from build123d import *

# Parameters (mm, degrees)
F0_W     = 160
F0_H     = 240
F0_R     = 3.25
F1_DEPTH = 6.35


# Not quite as in the source:
# - a length typed as a fraction of an inch, garbled in the dataset ("3 / 203.2 mm" for 3/8 in), is restored


with BuildPart() as f1:
    # F0 (on Top) → F1 (new body)
    with BuildSketch(Plane.XY):
        Rectangle(F0_W, F0_H)
        with Locations((-60, -100)):
            Circle(F0_R, mode=Mode.SUBTRACT)
        with Locations((-20, -100)):
            Circle(F0_R, mode=Mode.SUBTRACT)
        with Locations((-60, -60)):
            Circle(F0_R, mode=Mode.SUBTRACT)
        with Locations((-60, -20)):
            Circle(F0_R, mode=Mode.SUBTRACT)
        with Locations((-20, -60)):
            Circle(F0_R, mode=Mode.SUBTRACT)
        with Locations((-20, -20)):
            Circle(F0_R, mode=Mode.SUBTRACT)
        with Locations((20, -100)):
            Circle(F0_R, mode=Mode.SUBTRACT)
        with Locations((60, -100)):
            Circle(F0_R, mode=Mode.SUBTRACT)
        with Locations((20, -60)):
            Circle(F0_R, mode=Mode.SUBTRACT)
        with Locations((20, -20)):
            Circle(F0_R, mode=Mode.SUBTRACT)
        with Locations((60, -60)):
            Circle(F0_R, mode=Mode.SUBTRACT)
        with Locations((60, -20)):
            Circle(F0_R, mode=Mode.SUBTRACT)
        with Locations((-60, 20)):
            Circle(F0_R, mode=Mode.SUBTRACT)
        with Locations((-20, 20)):
            Circle(F0_R, mode=Mode.SUBTRACT)
        with Locations((-60, 60)):
            Circle(F0_R, mode=Mode.SUBTRACT)
        with Locations((-60, 100)):
            Circle(F0_R, mode=Mode.SUBTRACT)
        with Locations((-20, 60)):
            Circle(F0_R, mode=Mode.SUBTRACT)
        with Locations((-20, 100)):
            Circle(F0_R, mode=Mode.SUBTRACT)
        with Locations((20, 20)):
            Circle(F0_R, mode=Mode.SUBTRACT)
        with Locations((60, 20)):
            Circle(F0_R, mode=Mode.SUBTRACT)
        with Locations((20, 60)):
            Circle(F0_R, mode=Mode.SUBTRACT)
        with Locations((20, 100)):
            Circle(F0_R, mode=Mode.SUBTRACT)
        with Locations((60, 60)):
            Circle(F0_R, mode=Mode.SUBTRACT)
        with Locations((60, 100)):
            Circle(F0_R, mode=Mode.SUBTRACT)
    extrude(amount=F1_DEPTH)


solid = f1.part
Verification items for the finished model (mm, model axes). Round coordinates to 2 decimals unless told otherwise and drop trailing zeros. Loops run counter-clockwise (first coordinate to the right, second up) from the corner with the lowest first, then second, coordinate; pieces in that order, holes last. Notation, with made-up numbers: M 33,-34.5 L 42,-34.5 A20 ccw 42,-4.5 Z; hole C -1,27 d4. An arc over 180 degrees is marked long. Write each question's results on one line, items separated by ' | '.
1) Section check B-B on z = 1.5. State how many separate pieces and enclosed holes the cut face has, then the cut area to 3 significant figures.
Checks:
separate pieces: 1 | enclosed holes: 24 | area: 37,600 mm2
2) Section check A-A on x = -20. Record the boundary of the cut face in (y, z).
Checks:
outline: M -120,0 L -103.25,0 L -103.25,6.35 L -120,6.35 Z; M -96.75,0 L -63.25,0 L -63.25,6.35 L -96.75,6.35 Z; M -56.75,0 L -23.25,0 L -23.25,6.35 L -56.75,6.35 Z; M -16.75,0 L 16.75,0 L 16.75,6.35 L -16.75,6.35 Z; M 23.25,0 L 56.75,0 L 56.75,6.35 L 23.25,6.35 Z; M 63.25,0 L 96.75,0 L 96.75,6.35 L 63.25,6.35 Z; M 103.25,0 L 120,0 L 120,6.35 L 103.25,6.35 Z
3) Scan lines: L1, parallel to X at y = 57, z = 0.75; L2, parallel to X at y = 21, z = 5. Record each from-to range of solid material in increasing order. Write a range as from..to.
Checks:
L1: x = -80..-61.25, -58.75..-21.25, -18.75..18.75, 21.25..58.75, 61.25..80 | L2: x = -80..-63.09, -56.91..-23.09, -16.91..16.91, 23.09..56.91, 63.09..80
4) Gauge pin test, flat end, axial feed: P1, Ø5, axis at x = 60, y = -20, coming from the -Z side. Record the tip position at first contact, or that the pin passes through.
Checks:
P1: passes through
5) Mould release check, pull along Y, two halves, no side actions. Record for faces 1 (the cylindrical face through (-60.705, 96.827, 3.131)), 2 (the cylindrical face through (59.295, -103.173, 3.131)), 3 (the flat face through (-1, 2, 0)), 4 (the flat face through (-1, -120, 3)): released by +Y, released by -Y, zero draft, split by the parting line, or undercut.
Checks:
face 1: undercut | face 2: undercut | face 3: zero draft | face 4: released by -Y
6) Section check C-C on y = -20. Record the boundary of the cut face in (x, z).
Checks:
outline: M -80,0 L -63.25,0 L -63.25,6.35 L -80,6.35 Z; M -56.75,0 L -23.25,0 L -23.25,6.35 L -56.75,6.35 Z; M -16.75,0 L 16.75,0 L 16.75,6.35 L -16.75,6.35 Z; M 23.25,0 L 56.75,0 L 56.75,6.35 L 23.25,6.35 Z; M 63.25,0 L 80,0 L 80,6.35 L 63.25,6.35 Z
7) Section check D-D on x = 20.5. Record the boundary of the cut face in (y, z), then the cut area to 3 significant figures.
Checks:
outline: M -120,0 L -103.21,0 L -103.21,6.35 L -120,6.35 Z; M -96.79,0 L -63.21,0 L -63.21,6.35 L -96.79,6.35 Z; M -56.79,0 L -23.21,0 L -23.21,6.35 L -56.79,6.35 Z; M -16.79,0 L 16.79,0 L 16.79,6.35 L -16.79,6.35 Z; M 23.21,0 L 56.79,0 L 56.79,6.35 L 23.21,6.35 Z; M 63.21,0 L 96.79,0 L 96.79,6.35 L 63.21,6.35 Z; M 103.21,0 L 120,0 L 120,6.35 L 103.21,6.35 Z | area: 1,280 mm2
